Study the drawing (mm; zero at the part's minimum x, y, z) and answer. Coordinates: 2 decimals unless noted, no trailing zeros. Loops run counter-clockwise (first coordinate to the right, second up) from the corner with the lowest first, then second, coordinate; pieces in that order, holes last. Notation, with made-up numbers: (30.5, 21.5) - (35.5, 21.5) arc R27 ccw to (35.5, 57.5) - close; hole circle Ø6 at (-16.75, -22.75). An arc over 180 degrees is marked (long way). Write each question's results on one line, items separated by ' | '. Start each with the question number.
(1) Find section A-A on y = 6. Determine the outline of the cut face in (x, z).
(2) Consider line 1 (Y direction, x = 7, z = 1.15); line 2 (Y direction, x = 100, z = 0.8); line 3 (X direction, y = 6, z = 0.85). Determine where each line is inside the solid, lowest interval first. Write a range as from..to.
(3) Find section B-B on x = 100. Determine the outline of the cut face in (y, z), then the cut area to 3 significant figures.
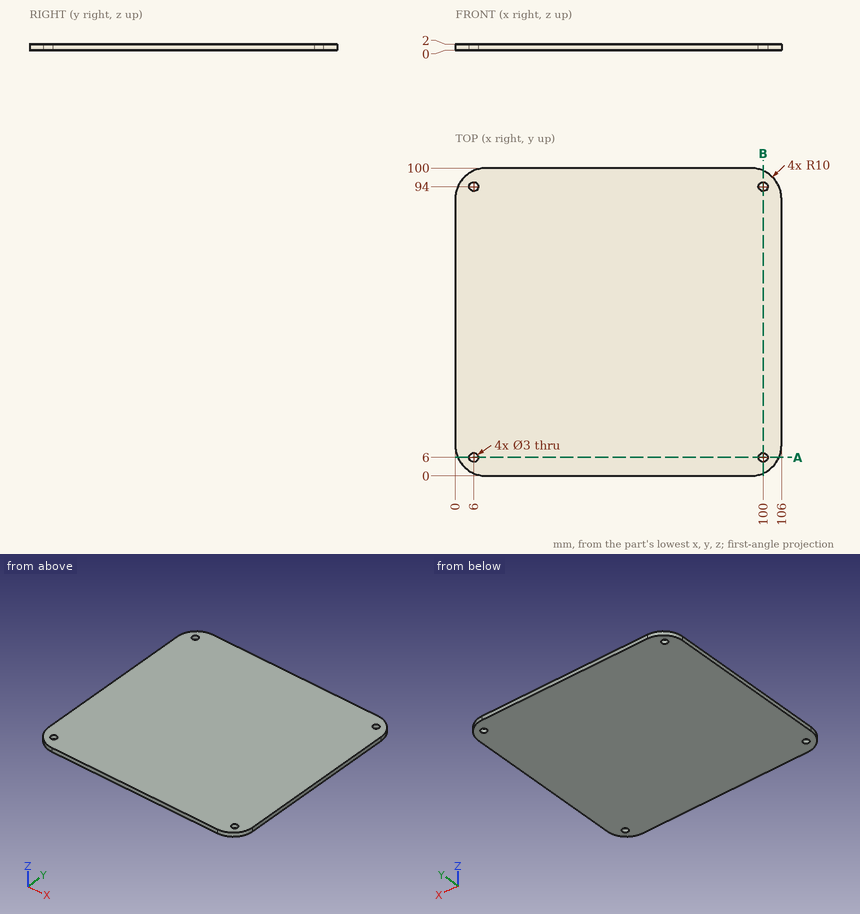
Values:
1) outline: (0.83, 0) - (4.5, 0) - (4.5, 2) - (0.83, 2) - close; (7.5, 0) - (98.5, 0) - (98.5, 2) - (7.5, 2) - close; (101.5, 0) - (105.17, 0) - (105.17, 2) - (101.5, 2) - close
2) line 1: y = 0.46..4.88, 7.12..92.88, 95.12..99.54 | line 2: y = 0.83..4.5, 7.5..92.5, 95.5..99.17 | line 3: x = 0.83..4.5, 7.5..98.5, 101.5..105.17
3) outline: (0.83, 0) - (4.5, 0) - (4.5, 2) - (0.83, 2) - close; (7.5, 0) - (92.5, 0) - (92.5, 2) - (7.5, 2) - close; (95.5, 0) - (99.17, 0) - (99.17, 2) - (95.5, 2) - close | area: 185 mm²
